Drawing for the job (mm, zero at the part's lowest x, y, z). Coordinates: 2 decimals unless noted, no trailing zeros. Write each loop counter-clockwise with the first axis right and the second up, starting at its lowest first coordinate (ties: lowest second). Pieces come first, ordered by that corner, then holes. Notation, with made-up numbers: (-9.75, 52) -> (20.25, 52) arc R19 cw to (20.25, 80) -> close; hole circle Ø2 at (12.25, 52.25). An arc over 180 degrees is marked (long way). Write item = value, one per line. Start each with the question number.
Q1. Band-saw the part on A-A, the plane z = 0.3. Give the number of separate pieces and of enclosed holes in the cut face, plus the area to 3 significant figures.
Q2. Probe line 1 (Y direction, x = 36.65, z = 0.9); line 2 (Y direction, x = 21.15, z = 0.75); line 3 (X direction, y = 36, z = 0.6). List the from-to ranges inside material, lowest first.
Q3. Band-saw the part on C-C, the plane x = 36.65. List the corners of the cut face in (y, z).
Q4. Band-saw the part on D-D, the plane x = 18. List the corners of the cut face in (y, z).
Q5. Band-saw the part on B-B, the plane y = 21.15. List the corners of the cut face in (x, z), plus the area to 3 significant figures.
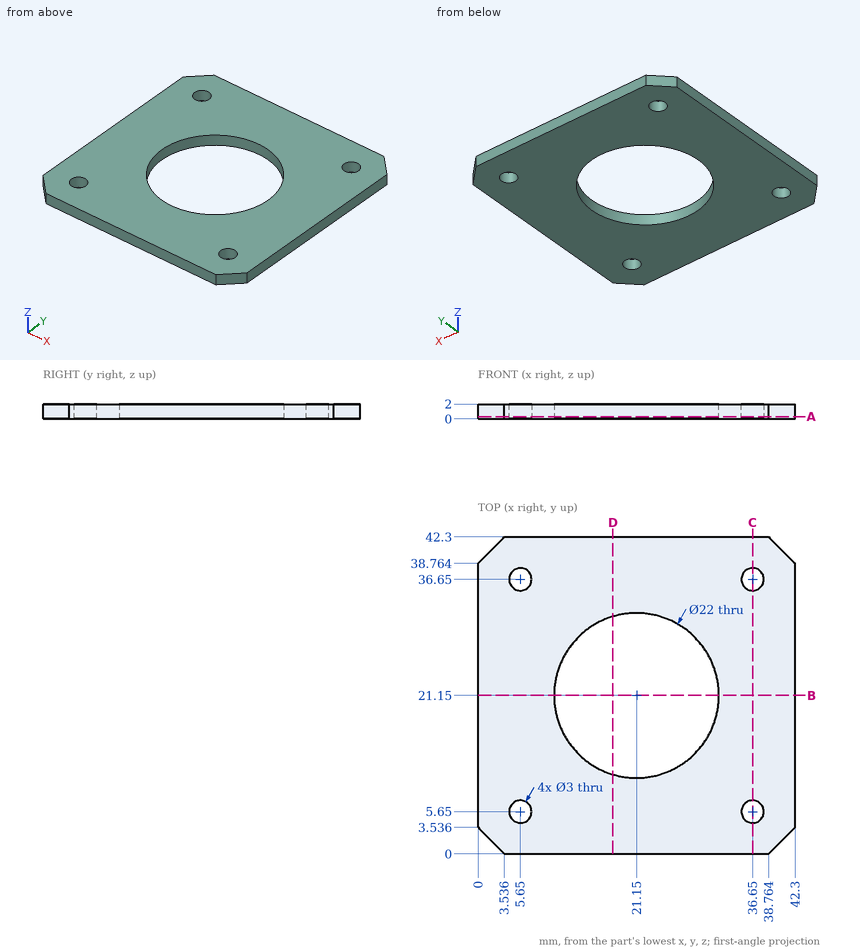
Ans:
q1.separate_pieces = 1
q1.enclosed_holes = 5
q1.area = 1,360 mm2
q2.line_1 = 0 to 4.15, 7.15 to 35.15, 38.15 to 42.3
q2.line_2 = 0 to 10.15, 32.15 to 42.3
q2.line_3 = 0 to 4.3, 7 to 35.3, 38 to 42.3
q3.outline = (0, 0) -> (4.15, 0) -> (4.15, 2) -> (0, 2) -> close; (7.15, 0) -> (35.15, 0) -> (35.15, 2) -> (7.15, 2) -> close; (38.15, 0) -> (42.3, 0) -> (42.3, 2) -> (38.15, 2) -> close
q4.outline = (0, 0) -> (10.61, 0) -> (10.61, 2) -> (0, 2) -> close; (31.69, 0) -> (42.3, 0) -> (42.3, 2) -> (31.69, 2) -> close
q5.outline = (0, 0) -> (10.15, 0) -> (10.15, 2) -> (0, 2) -> close; (32.15, 0) -> (42.3, 0) -> (42.3, 2) -> (32.15, 2) -> close
q5.area = 40.6 mm2
